```python
from build123d import *

# Parameters (mm, degrees)
BOSS_EXTRUDE2_DEPTH = 15.24
SKETCH3_R           = 12.099925
SKETCH3_R_2         = 10.715625
BOSS_EXTRUDE3_DEPTH = 19.05


with BuildPart() as part:
    # Sketch1 → Boss-Extrude2 (new, symmetric)
    with BuildSketch(Plane.XY):
        with BuildLine():
            Line((-31.75, 10.715625), (31.75, 10.715625))
            ThreePointArc((31.75, 10.715625), (21.034375, 0), (31.75, -10.715625))
            Line((31.75, -10.715625), (-31.75, -10.715625))
            ThreePointArc((-31.75, -10.715625), (-21.034375, 0), (-31.75, 10.715625))
        make_face()
    extrude(amount=BOSS_EXTRUDE2_DEPTH, both=True)

    # Sketch3 → Boss-Extrude3 (add)
    with BuildSketch(Plane(origin=(0, 10.715625, 0), x_dir=(1, 0, 0), z_dir=(0, 1, 0))):
        Circle(SKETCH3_R)
        Circle(SKETCH3_R_2, mode=Mode.SUBTRACT)
    extrude(amount=BOSS_EXTRUDE3_DEPTH)


solid = part.part
```
Work out the finished part from the listing and answer in its coordinate system (mm). A direction names the side the tool comes from. Round coordinates to 2 decimals unless told otherwise and drop trailing zeros. Loops run counter-clockwise (first coordinate to the right, second up) from the corner with the lowest first, then second, coordinate; pieces in that order, holes last. Notation, with made-up numbers: M -26.5,-10.75 L 16.5,-10.75 A13 ccw 16.5,-0.75 Z; hole C 66,-4 d5. An arc over 180 degrees is marked long. Use CSV: the item, a comma, the result in double quotes.
Q1. The mould has two halves that part along Y. Classify faces 3 (the flat face through (0, -10.716, 0)), 4 (the cylindrical face through (21.037, 0.236, 0.213)), 5 (the cylindrical face through (-21.037, -0.236, 0.213)), 6 (the flat face through (-1, 29.766, 11)): pulls with the +Y half, pulls with the -Y half, needs draft (parallel to the pull), parting line crosses it, or undercut.
Determined:
face 3,"pulls with the -Y half"
face 4,"undercut"
face 5,"undercut"
face 6,"pulls with the +Y half"
Q2. Section A-A, the plane x = 0 is taken. Determine the outline of the cut face in (y, z).
Determined:
outline,"M -10.72,-15.24 L 10.72,-15.24 L 10.72,-12.1 L 29.77,-12.1 L 29.77,-10.72 L 10.72,-10.72 L 10.72,10.72 L 29.77,10.72 L 29.77,12.1 L 10.72,12.1 L 10.72,15.24 L -10.72,15.24 Z"
Q3. A tool of negligible diameter and unlimited length cuts with its end or side. For faces 1 (the flat face through (0, 0, 15.24)), 2 (the flat face through (0, 10.716, 0)), from which of +Z, -Z, +X, -X, +Y, -Y can it reach the whole face along a straight path? Write none if from no direction.
Determined:
face 1,"+Z, +X, -X, +Y, -Y"
face 2,"+Y"
Q4. Section C-C, the plane x = 26 is taken. Determine the outline of the cut face in (y, z), then the cut area to 3 significant figures.
Determined:
outline,"M -10.72,-15.24 L -9.04,-15.24 L -9.04,15.24 L -10.72,15.24 Z; M 9.04,-15.24 L 10.72,-15.24 L 10.72,15.24 L 9.04,15.24 Z"
area,"102 mm2"
Q5. Each of these flat-tipped pins is pushed along its axis until it touches: pin 1 (1 mm diameter, centred on x = -16, z = -11.5, fed in from +Y); pin 2 (3 mm diameter, centred on y = 6, z = -2.5, fed in from -X); pin 3 (2 mm diameter, centred on y = 18, z = 0, fed in from +X). Where does it stop, or does it pass through?
Determined:
pin 1,"y = 10.72"
pin 2,"x = -24.1"
pin 3,"x = 12.1"
Q6. Consider L1, parallel to X at y = 23.25, z = 0; L2, parallel to Y at x = 4, z = 1. Determine where each line is inside the solid, lowest interval first.
Determined:
L1,"-12.1 to -10.72, 10.72 to 12.1"
L2,"-10.72 to 10.72"
Q7. Section B-B, the plane z = -4 is taken. Determine the outline of the cut face in (x, y), then the cut area to 3 significant figures.
Determined:
outline,"M -31.75,-10.72 L 31.75,-10.72 A10.72 cw 31.75,10.72 L 11.42,10.72 L 11.42,29.77 L 9.94,29.77 L 9.94,10.72 L -9.94,10.72 L -9.94,29.77 L -11.42,29.77 L -11.42,10.72 L -31.75,10.72 A10.72 cw Z"
area,"1,060 mm2"
Q8. Section D-D, the plane y = 27.5 is taken. Determine the outline of the cut face in (x, z), then the cut area to 3 significant figures.
Determined:
outline,"C 0,0 d24.2; hole C 0,0 d21.43"
area,"99.2 mm2"
